```python
from build123d import *

# Parameters (mm, degrees)
F0_R          = 12.75
F0_R_2        = 3.25
F1_DEPTH      = 5
F0_R_3        = 20
F2_DEPTH      = 6
F2_DEPTH_BACK = 5
F3_SIZE       = 5
F4_R          = 16
F5_DEPTH      = 3
F6_START      = 4
F6_DEPTH      = 21
F7_R          = 16.5
F7_R_2        = 12.7
F8_DEPTH      = 4
F8_DEPTH_BACK = 5


with BuildPart() as f1:
    # F0 (on Top) → F1 (new body)
    with BuildSketch(Plane.XY):
        Circle(F0_R)
        Circle(F0_R_2, mode=Mode.SUBTRACT)
    extrude(amount=F1_DEPTH)

    # F0 (on Top) → F2 (join, two sides)
    with BuildSketch(Plane.XY) as f2_sk:
        Circle(F0_R_3)
        Circle(F0_R, mode=Mode.SUBTRACT)
    extrude(amount=F2_DEPTH)
    extrude(f2_sk.sketch, amount=-F2_DEPTH_BACK)

    # F3
    f3_edges = [f1.edges().sort_by_distance(p)[0] for p in [
        (-20, 0, -5),
    ]]
    chamfer(f3_edges, length=F3_SIZE)

    # F4 (on Top) → F5 (cut)
    with BuildSketch(Plane.XY):
        Circle(F4_R)
    extrude(amount=F5_DEPTH, mode=Mode.SUBTRACT)

    # F4 (on Top) → F6 (cut)
    with BuildSketch(Plane.XY.offset(F6_START)):
        Circle(F4_R)
    extrude(amount=F6_DEPTH, mode=Mode.SUBTRACT)

    # F7 (on Top) → F8 (join, two sides)
    with BuildSketch(Plane.XY) as f8_sk:
        Circle(F7_R)
        Circle(F7_R_2, mode=Mode.SUBTRACT)
    extrude(amount=F8_DEPTH)
    extrude(f8_sk.sketch, amount=-F8_DEPTH_BACK)


solid = f1.part
```
Can you work these out from the model? Positions are in its coordinate system, mm. A direction names the side the tool comes from. Coordinates: 2 decimals unless noted, no trailing zeros. Order: outer loops, then holes, each group sorted by start corner. A loop starts at its lowest first (then second) coordinate and runs counter-clockwise, first axis right, second up. Notation, with made-up numbers: (79.25, -1) - (92.25, -1) arc R10 cw to (92.25, 3) - close; hole circle Ø11 at (-9.75, 74.5). An arc over 180 degrees is marked (long way). Answer in a Markdown table with one row per item.
1. Suppose I cut it at A-A (x = 0). Please give me the cut outline in (y, z).
Reply:
| item | result |
|---|---|
| outline | (-20, 0) - (-16.5, -3.5) - (-16.5, -5) - (-12.7, -5) - (-12.7, 3) - (-3.25, 3) - (-3.25, 4) - (-16, 4) - (-16, 6) - (-20, 6) - close; (3.25, 3) - (12.7, 3) - (12.7, -5) - (16.5, -5) - (16.5, -3.5) - (20, 0) - (20, 6) - (16, 6) - (16, 4) - (3.25, 4) - close |
2. If we mould it in two halves opening along X, with no side actions, what happens to faces 1 (the conical face through (15.9, 5.01, -3.33)), 2 (the cylindrical face through (-2.579, -1.978, 3.493)), 3 (the flat face through (8.5, -9.7, -5)), 4 (the cylindrical face through (-2.75, -12.4, -0.94))? For each: pulls with the +X half, pulls with the -X half, needs draft (parallel to the pull), parting line crosses it, or undercut.
Reply:
| item | result |
|---|---|
| face 1 | parting line crosses it |
| face 2 | undercut |
| face 3 | needs draft |
| face 4 | undercut |
3. For faces 5 (the cylindrical face through (-3.47, -15.62, 4.99)), 6 (the cylindrical face through (-3.577, -16.108, -4.24)), 7 (the cylindrical face through (-4.336, -19.524, 3.042)), which set-ups out of +Z, -Z, +X, -X, +Y, -Y let a thin tool reach every point of the face, with its end or its side?
Reply:
| item | result |
|---|---|
| face 5 | +Z |
| face 6 | -Z |
| face 7 | +Z, -Z |
4. If I drill on line 1 along Y through (x, z) = (0, 5.35); line 2 along Y through (x, z) = (0, 1); line 3 along X through (y, z) = (11, 4.75), over which ranges is the centre line in solid material (lowest first)?
Reply:
| item | result |
|---|---|
| line 1 | y = -20 to -16, 16 to 20 |
| line 2 | y = -20 to -12.7, 12.7 to 20 |
| line 3 | x = -16.7 to -11.62, 11.62 to 16.7 |
5. Suppose I cut it at D-D (z = -2.25). Please give me the cut outline in (x, y).
Reply:
| item | result |
|---|---|
| outline | circle Ø35.5 at (0, 0); hole circle Ø25.4 at (0, 0) |
6. For pin 1 (3 mm diameter, centred on x = -4.5, z = 3.5, fed in from -Y); pin 2 (4 mm diameter, centred on x = 4.5, z = 3.5, fed in from +Y); pin 3 (5 mm diameter, centred on y = 15, z = -0.5, fed in from -X); pin 4 (4 mm diameter, centred on x = 0, y = 0, fed in from -Z), each with a flat end and sliding along its axis, tell me the tip position at first contact or that it passes through.
Reply:
| item | result |
|---|---|
| pin 1 | stops at y = -19.77 |
| pin 2 | stops at y = 19.84 |
| pin 3 | stops at x = -15.57 |
| pin 4 | passes through |
7. Suppose I cut it at C-C (z = 2.25). Please give me the cut outline in (x, y), and give its area (3 significant figures).
Reply:
| item | result |
|---|---|
| outline | circle Ø40 at (0, 0); hole circle Ø25.4 at (0, 0) |
| area | 750 mm^2 |
